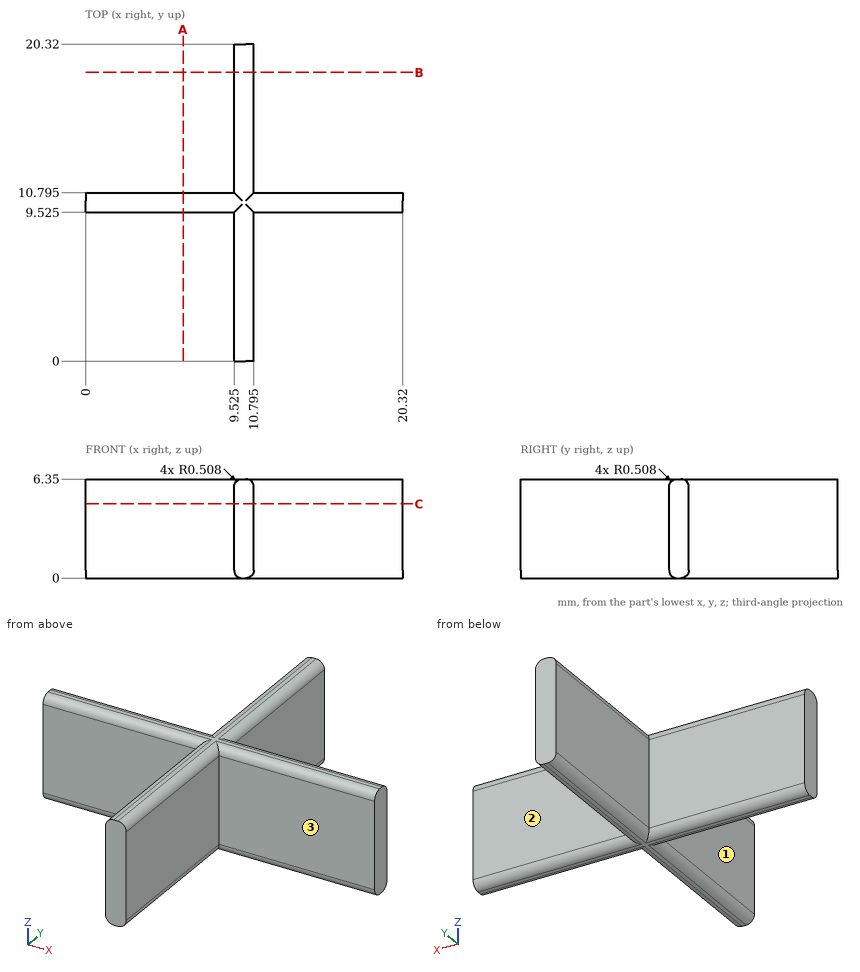
Can you work these out from the drawing? Everything is in mm from the part's minimum corner. A direction names the side the tool comes from. Coordinates: 2 decimals unless noted, no trailing zeros. Loops run counter-clockwise (first coordinate to the right, second up) from the corner with the lowest first, then second, coordinate; pieces in that order, holes last. Notation, with made-up numbers: (-5.75, 68) - (22.25, 68) arc R21 ccw to (22.25, 73) - close; hole circle Ø3 at (-28, 79). An arc over 180 degrees is marked (long way). Put each result on its own line as item: value. Start each with the question number.
Item 1: Which directions (+Z, -Z, +X, -X, +Y, -Y) give clear straight access to the entire face, cutting with the end or side of a thin tool? Please do the marked faces 1, 2 and 3.
Item 2: For pin 1 (1.5 mm diameter, centred on x = 6, z = 3.5, fed in from +Y) (3 decimals); pin 2 (2 mm diameter, centred on x = 12.5, z = 5, fed in from -Y) (3 decimals), each with a flat end and sliding along its axis, tell me the tip position at first contact or that it passes through.
Item 3: Suppose I cut it at C-C (z = 4.75). Please give me the cut outline in (x, y) (3 decimals), and give its area (3 significant figures).
Item 4: If I drill on line 1 along X through (y, z) = (7.75, 4) (3 decimals); line 2 along Y through (x, z) = (1, 6.25), over which ranges is the centre line in solid material (lowest first)?
Item 5: Suppose I cut it at A-A (x = 6.25). Please give me the cut outline in (y, z) (3 decimals).
Here are the results:
1. face 1: +Z, -Z, -X, -Y
1. face 2: +Z, -Z, +X, +Y
1. face 3: +Z, -Z, +X, -Y
2. pin 1: y = 10.795
2. pin 2: y = 9.525
3. outline: (0, 9.525) - (9.525, 9.525) - (9.525, 0) - (10.795, 0) - (10.795, 9.525) - (20.32, 9.525) - (20.32, 10.795) - (10.795, 10.795) - (10.795, 20.32) - (9.525, 20.32) - (9.525, 10.795) - (0, 10.795) - close
3. area: 50.0 mm²
4. line 1: 9.525 to 10.795
4. line 2: 9.73 to 10.59
5. outline: (9.525, 0.508) arc R0.508 ccw to (10.033, 0) - (10.287, 0) arc R0.508 ccw to (10.795, 0.508) - (10.795, 5.842) arc R0.508 ccw to (10.287, 6.35) - (10.033, 6.35) arc R0.508 ccw to (9.525, 5.842) - close
